Source: three-view drawing plus pictorial views. Frame: mm from the lowest corner of the part. A direction names the side the tool comes from. Coordinates: 2 decimals unless noted, no trailing zeros. Loops run counter-clockwise (first coordinate to the right, second up) from the corner with the lowest first, then second, coordinate; pieces in that order, holes last. Notation, with made-up numbers: M -9,-28 L -5,-28 A25 ccw -5,8 Z; hole C 55,29.25 d4. An arc over 180 degrees is marked long. Use a Markdown table: item, result. Add a question column.
1. Section A-A on y = 36. Output: boundary loops of the cut face in (x, z) (3 decimals), then the cut area to 3 significant figures.
2. Draft query along Z for the marked faces 3, 4 and 5. Return one class per face: +Z half, -Z half, draft (parallel to the pull), parting line (faces both ways), or undercut.
3. Line query: L1, parallel to Z at x = 20.5, y = 21.5 (3 decimals); L2, parallel to X at y = 11.5, z = 45 (3 decimals); L3, parallel to Y at x = 15, z = 71. Output: solid intervals per line, ascending. Write a range as [from, to].
4. Set-up query: the marked faces 1 and 2. Return all of +Z, -Z, +X, -X, +Y, -Y with unobstructed straight access to the full face (end or side cutting, diameter ignored); none if empty.
5. Pin query (flat end, axial travel): pin 1 (5 mm diameter, centred on y = 31.5, z = 55.5, fed in from -X); pin 2 (8 mm diameter, centred on x = 8.5, z = 32, fed in from +Y). Return the tip coordinate at first contact, or that it passes through.
6. Section C-C on z = 70. Output: boundary loops of the cut face in (x, y) (3 decimals), then the cut area to 3 significant figures.
7. Section B-B on x = 48. Output: boundary loops of the cut face in (y, z) (3 decimals).
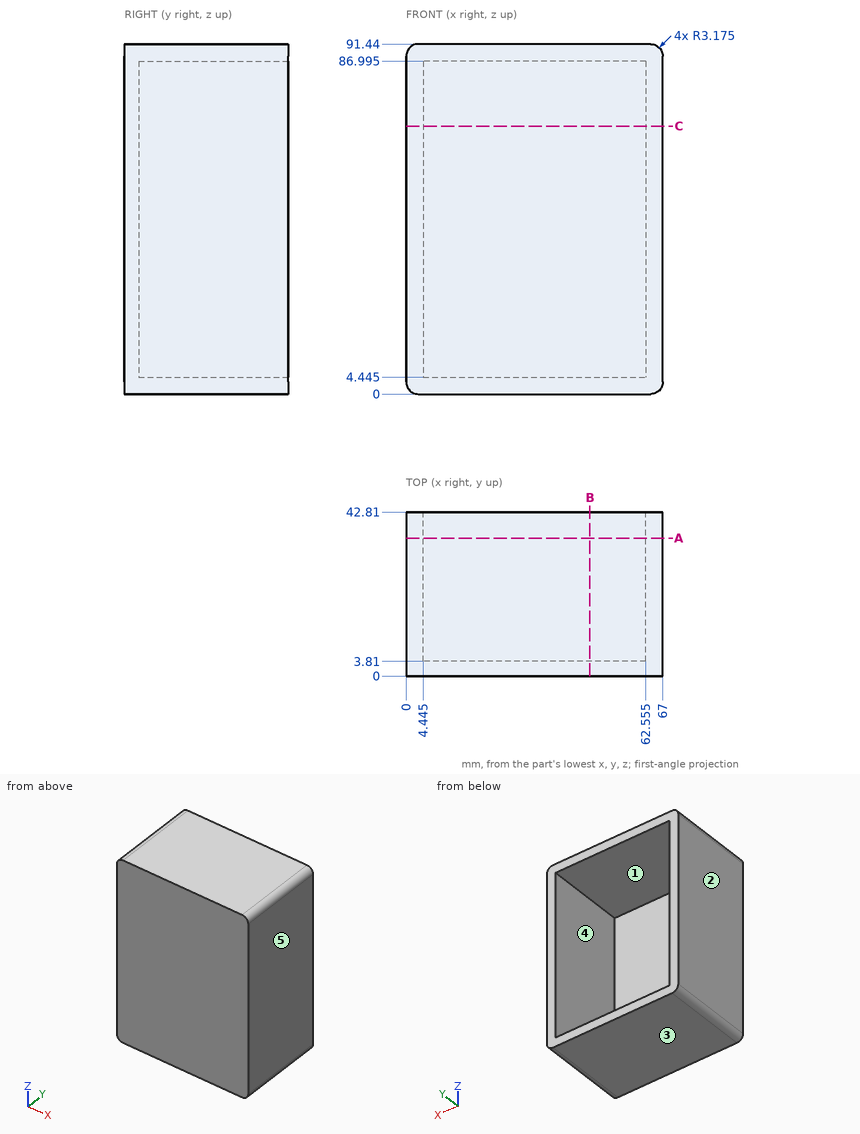
Answers below:
| question | item | result |
|---|---|---|
| 1 | outline | M 0,3.175 A3.175 ccw 3.175,0 L 63.825,0 A3.175 ccw 67,3.175 L 67,88.265 A3.175 ccw 63.825,91.44 L 3.175,91.44 A3.175 ccw 0,88.265 Z; hole M 4.445,4.445 L 62.555,4.445 L 62.555,86.995 L 4.445,86.995 Z |
| 1 | area | 1,320 mm² |
| 2 | face 3 | -Z half |
| 2 | face 4 | undercut |
| 2 | face 5 | draft |
| 3 | L1 | z = [0, 4.445], [86.995, 91.44] |
| 3 | L2 | x = [0, 4.445], [62.555, 67] |
| 3 | L3 | y = [0, 3.81] |
| 4 | face 1 | +Y |
| 4 | face 2 | +Z, -Z, -X, +Y, -Y |
| 5 | pin 1 | stops at x = 0 |
| 5 | pin 2 | stops at y = 3.81 |
| 6 | outline | M 0,0 L 67,0 L 67,42.81 L 62.555,42.81 L 62.555,3.81 L 4.445,3.81 L 4.445,42.81 L 0,42.81 Z |
| 6 | area | 602 mm² |
| 7 | outline | M 0,0 L 42.81,0 L 42.81,4.445 L 3.81,4.445 L 3.81,86.995 L 42.81,86.995 L 42.81,91.44 L 0,91.44 Z |
